Read the model definition and answer for the solid it produces. Units are mm, in the model's axes. A direction names the side the tool comes from. Coordinates: 2 decimals unless noted, no trailing zeros. Order: outer loops, then holes, each group sorted by start corner. A loop starts at its lowest first (then second) coordinate and runs counter-clockwise, first axis right, second up.
Autodesk Inventor part; units mm, degrees
ref_plane "YZ Plane" through (0, 0, 0) normal (1, 0, 0) x (0, 1, 0)
ref_plane "XZ Plane" through (0, 0, 0) normal (0, 1, 0) x (-1, 0, 0)
ref_plane "XY Plane" through (0, 0, 0) normal (0, 0, 1) x (1, 0, 0)
sketch "Sketch1" plane through (0, 0, 0) normal (0, 1, 0) x (-1, 0, 0)
  line L0 (0, 0) -> (0, 23.8143)
  line L1 (0, 23.8143) -> (7.4151, 29.5041)
  line L2 (0, 23.8143) -> (9.3465, 23.8143) construction
  line L3 (0, 23.8143) -> (28, 45.2994)
  line L4 (0, 23.8143) -> (0, -23.8137)
  line L5 (0, -23.8137) -> (28, -45.2989)
  line L6 (28, -45.2989) -> (26.4781, -47.2823)
  line L7 (26.4781, -47.2823) -> (-0.4066, -26.6529)
  line L8 (0, -16.592) -> (-2.5, -16.592)
  line L9 (-2.5, -16.592) -> (-2.5, -25.0466)
  line L10 (-2.5, -25.0466) -> (-0.4066, -26.6529)
  line L11 (-2.5, -16.592) -> (-2.5, 22.9887)
  line L12 (0.8654, 24.4783) -> (-0.6565, 26.4617)
  line L13 (-0.6565, 26.4617) -> (-2.5, 25.0471)
  line L14 (-2.5, 25.0471) -> (-2.5, 22.9887)
  line L15 (-0.6565, 26.4617) -> (26.4781, 47.2828)
  line L16 (26.4781, 47.2828) -> (28, 45.2994)
  line L17 (26.4781, 47.2828) -> (28, 45.2994)
  line L18 (28, 45.2994) -> (0.8654, 24.4783)
  dimension "d0" = 23.8143
  dimension "d1" = 37.5
  dimension "d2" = 35.2932
  dimension "d3" = 47.628
  dimension "d4" = 35.2932
  dimension "d5" = 2.5
  dimension "d6" = 2.5
  dimension "d7" = 2.5
extrude "Extrusion1" add sketch "Sketch1" along normal blind 40
sketch "Sketch2" plane through (0, 40, 0) normal (0, 1, 0) x (1, 0, 0)
  line L0 (0, 0) -> (8, 0)
  line L1 (-28, 45.2989) -> (0, 23.8137)
  line L2 (-28, 45.2989) -> (-24.0332, 42.2551)
  line L3 (-24.0332, 42.2551) -> (-19.1631, 48.6019)
  line L4 (0, -23.8143) -> (-28, -45.2994)
  line L5 (-28, -45.2994) -> (-24.0332, -42.2556)
  line L6 (-24.0332, -42.2556) -> (-19.1631, -48.6024)
  circle A0 centre (-19.1631, -48.6024) radius 1.75
  circle A1 centre (-19.1631, -48.6024) radius 3.5
  circle A2 centre (8, 0) radius 1.75
  circle A3 centre (8, 0) radius 3.5
  circle A4 centre (-19.1631, 48.6019) radius 1.75
  circle A5 centre (-19.1631, 48.6019) radius 3.5
  line L7 (2.5, 25.0466) -> (-26.4781, 47.2823)
  line L8 (-22.5113, 44.2385) -> (-25.2881, 46.3691)
  line L9 (-25.2881, 46.3691) -> (-21.9399, 50.7326)
  line L10 (-22.5113, 44.2385) -> (-19.7346, 42.1078)
  line L11 (-19.7346, 42.1078) -> (-16.3864, 46.4712)
  line L12 (8, 3.5) -> (2.5, 3.5)
  line L13 (2.5, 3.5) -> (2.5, -3.5)
  line L14 (2.5, -25.0471) -> (2.5, 25.0466)
  line L15 (2.5, -3.5) -> (8, -3.5)
  line L16 (-26.4781, -47.2828) -> (2.5, -25.0471)
  line L17 (-22.5113, -44.239) -> (-19.7346, -42.1083)
  line L18 (-19.7346, -42.1083) -> (-16.3864, -46.4718)
  line L19 (-22.5113, -44.239) -> (-25.2881, -46.3697)
  line L20 (-25.2881, -46.3697) -> (-21.9399, -50.7331)
  dimension "d10" = 8
  dimension "d11" = 5
  dimension "d12" = 8
  dimension "d13" = 8
  dimension "d14" = 3.5
  dimension "d15" = 7
  dimension "d16" = 3.5
  dimension "d17" = 7
  dimension "d18" = 3.5
  dimension "d19" = 7
  dimension "d20" = 3.5
  dimension "d21" = 3.5
extrude "Extrusion2" add sketch "Sketch2" against normal blind 3
sketch "Sketch3" plane through (0, 0, 0) normal (0, -1, 0) x (1, 0, 0)
  line L0 (0, 0) -> (0, 10)
  line L1 (0, -23.8137) -> (0, 23.8143)
  line L2 (0, 10) -> (0, -10)
  line L3 (0, -10) -> (8, -10)
  line L4 (0, 10) -> (8, 10)
  circle A0 centre (8, 10) radius 1.75
  circle A1 centre (8, -10) radius 1.75
  circle A2 centre (8, -10) radius 3.5
  circle A3 centre (8, 10) radius 3.5
  line L5 (2.5, 25.0471) -> (2.5, -25.0466)
  line L6 (2.5, 10) -> (2.5, 6.5)
  line L7 (2.5, 6.5) -> (8, 6.5)
  line L8 (2.5, 10) -> (2.5, 13.5)
  line L9 (2.5, 13.5) -> (8, 13.5)
  line L10 (2.5, -10) -> (2.5, -13.5)
  line L11 (2.5, -13.5) -> (8, -13.5)
  line L12 (2.5, -10) -> (2.5, -6.5)
  line L13 (2.5, -6.5) -> (8, -6.5)
  dimension "d24" = 10
  dimension "d25" = 20
  dimension "d26" = 8
  dimension "d27" = 3.5
  dimension "d28" = 7
extrude "Extrusion3" add sketch "Sketch3" against normal blind 3 contours L5 L9 A3 L4 | L4 A3 L7 L5 | L5 L13 A2 L3 | L3 A2 L11 L5 | A3 | A2
sketch "Sketch4" plane through (0, 0, 0) normal (0, -1, 0) x (1, 0, 0)
  line L0 (2.5, 13.5) -> (8, 13.5)
  line L1 (2.5, 13.5) -> (12.0473, 13.5)
  line L2 (12.0473, 13.5) -> (12.0473, 6.5)
  line L3 (12.0473, 6.5) -> (2.5, 6.5)
  line L4 (2.5, 6.5) -> (2.5, 13.5)
  line L5 (2.5, -6.5) -> (8, -6.5)
  line L6 (2.5, -6.5) -> (13.899, -6.5)
  line L7 (13.899, -6.5) -> (13.899, -13.5)
  line L8 (13.899, -13.5) -> (2.5, -13.5)
  line L9 (2.5, -13.5) -> (2.5, -6.5)
  point P0 (0, 0)
  dimension "d31" = 7
extrude "Extrusion4" cut sketch "Sketch4" against normal blind 3
sketch "Sketch5" plane through (0, 0, 0) normal (0, -1, 0) x (1, 0, 0)
  point P0 (0, 0)
fillet "Fillet1" radius 20 4 edges at (0, 20, -23.8137) (0, 20, 23.8143) (2.5, 20, 25.0471) (2.5, 20, -25.0466)
sketch "Sketch6" plane through (0, 0, 0) normal (0, -1, 0) x (1, 0, 0)
  line L0 (0, 0) -> (0, 10)
  line L1 (0, -13.9508) -> (0, 13.9514)
  line L2 (0, 10) -> (8, 10)
  circle A0 centre (8, 10) radius 1.75
  circle A1 centre (8, 10) radius 3.5
  line L3 (2.5, 15.1842) -> (2.5, 3.5)
  line L4 (2.5, 10) -> (2.5, 13.5)
  line L5 (2.5, 13.5) -> (8, 13.5)
  line L6 (2.5, 10) -> (2.5, 6.5)
  line L7 (2.5, 6.5) -> (8, 6.5)
  line L8 (0, 0) -> (0, -10)
  line L9 (0, -10) -> (8, -10)
  circle A2 centre (8, -10) radius 1.75
  circle A3 centre (8, -10) radius 3.5
  line L10 (8, -6.5) -> (2.5, -6.5)
  line L11 (2.5, 15.1842) -> (2.5, -15.1837)
  line L12 (2.5, -6.5) -> (2.5, -13.5)
  line L13 (2.5, -13.5) -> (8, -13.5)
  dimension "d35" = 10
  dimension "d36" = 8
  dimension "d37" = 3.5
  dimension "d38" = 7
  dimension "d39" = 10
  dimension "d40" = 8
extrude "Extrusion5" add sketch "Sketch6" against normal blind 3 contours L3 L5 A1 L2 | L2 A1 L7 L3 | L11 L10 A3 L9 | L9 A3 L13 L11 | A1 | A3
properties part number "Capcture Zone4"
1) A cutting plane is placed at B-B, the plane x = -13.5. Determine the outline of the cut face in (y, z).
A:
outline: (0, -37.32) - (40, -37.32) - (40, -34.17) - (0, -34.17) - close; (0, 34.17) - (40, 34.17) - (40, 37.32) - (0, 37.32) - close
2) A cutting plane is placed at C-C, the plane z = 39. Determine the outline of the cut face in (x, y), and give its area (3 significant figures).
A:
outline: (-19.79, 0) - (-15.68, 0) - (-15.68, 40) - (-19.79, 40) - close
area: 164 mm2
3) Which of the six approach directions +Z, -Z, +X, -X, +Y, -Y give full straight-line access (tool end or side, diameter ignored) to faces 1 (the flat face through (-18.084, 38.521, 44.26)), 2 (the flat face through (6, 3, -10)), 3 (the flat face through (-17.77, 19.72, 37.45)), 4 (the flat face through (-23.64, 38.52, 48.52)), 5 (the flat face through (-21, 37, 47))?
A:
face 1: +X, +Y, -Y
face 2: +Z, -Z, +X, +Y
face 3: -X, +Y, -Y
face 4: +Z, +Y, -Y
face 5: +Z, +X, -Y
4) Flat-ended cylindrical pins translate along their axes: pin 1 Ø2 at (x, y) = (-22, 5.5) entering from +Z; pin 2 Ø5 at (x, z) = (-22.5, -45.5) entering from -Y; pin 3 Ø1.5 at (x, y) = (6, 1.5) entering from -Z; pin 4 Ø3 at (x, y) = (-20.5, 15) entering from -Z. Find the tip coordinate at first contact, or state that the pin passes through.
A:
pin 1: stops at z = 44.61
pin 2: stops at y = 0
pin 3: stops at z = -13.5
pin 4: stops at z = -43.85
5) Determine the mould class of faces 6 (the flat face through (5, 39, -3.5)), 7 (the cylindrical face through (-2.006, 20.28, -22.681)), 8 (the cylindrical face through (11.5, 1.5, 9.9)), 9 (the flat face through (5, 1, 13.5)) for opening direction Z: pulls with the +Z half, pulls with the -Z half, needs draft (parallel to the pull), parting line crosses it, or undercut.
A:
face 6: pulls with the -Z half
face 7: undercut
face 8: undercut
face 9: pulls with the +Z half
6) A cutting plane is placed at A-A, the plane z = 10. Determine the outline of the cut face in (x, y).
A:
outline: (0, 0) - (6.25, 0) - (6.25, 3) - (2.5, 3) - (2.5, 40) - (0, 40) - close; (9.75, 0) - (11.5, 0) - (11.5, 3) - (9.75, 3) - close
7) Straight lines are drawn through the part: line 1 (Z direction, x = 8, y = 2); line 2 (X direction, y = 38.35, z = 0); line 3 (X direction, y = 36.5, z = 0). For each, find the intervals that lie inside material, in ascending order.
A:
line 1: z = -13.5 to -11.75, -8.25 to -6.5, 6.5 to 8.25, 11.75 to 13.5
line 2: x = 0 to 6.25, 9.75 to 11.5
line 3: x = 0 to 2.5
